Source: CAD feature listing. Evaluate the final solid. Frame: model axes, mm. Give positions to 0.01 mm unless a question says otherwise; leave off trailing zeros. Loops run counter-clockwise (first coordinate to the right, second up) from the corner with the lowest first, then second, coordinate; pieces in that order, holes last. Notation, with made-up numbers: (-22.75, 7) -> (31.25, 7) arc R14 ccw to (31.25, 11) -> close; hole circle Ø4 at (81, 82.25). An arc over 180 degrees is marked (long way). Return JSON: item names as keys, results as strings. Group by question number.
(1) Cut plane C-C on y = 2. Return loops of the section in (x, z).
(2) Cut plane A-A on x = -36. Return loops of the section in (y, z).
(3) Cut plane B-B on z = 0.2. Return loops of the section in (x, y).
(4) Ray query, line 1 (Y direction, x = -37, z = 0.6); line 2 (X direction, y = 8, z = -0.65). Return the intervals inside material, ascending. Write a range as from..to.
(5) Pin query (flat end, axial travel): pin 1 (0.6 mm diameter, centred on y = 3, z = -0.5, fed in from -X). Return the tip coordinate at first contact, or that it passes through.
```python
from build123d import *

# Parameters (mm, degrees)
F1_DEPTH = 1


with BuildPart() as f1:
    # F0 (on Top) → F1 (new body, symmetric)
    with BuildSketch(Plane.XY):
        Polygon((-50, -50), (50, -50), (50, 50), (-50, 50), (-50, 11), (-30, 11), (-30, -11), (-50, -11), align=None)
    extrude(amount=F1_DEPTH, both=True)


solid = f1.part
```
Answers:
{
 "1": {"outline": "(-30, -1) -> (50, -1) -> (50, 1) -> (-30, 1) -> close"},
 "2": {"outline": "(-50, -1) -> (-11, -1) -> (-11, 1) -> (-50, 1) -> close; (11, -1) -> (50, -1) -> (50, 1) -> (11, 1) -> close"},
 "3": {"outline": "(-50, -50) -> (50, -50) -> (50, 50) -> (-50, 50) -> (-50, 11) -> (-30, 11) -> (-30, -11) -> (-50, -11) -> close"},
 "4": {"line 1": "-50..-11, 11..50", "line 2": "-30..50"},
 "5": {"pin 1": "x = -30"}
}
